Design review of the part shown in the three views and the two pictorial views. Dimensions are in mm from the part's minimum x, y and z. Give positions to 0.01 mm unless a question says otherwise; leave off trailing zeros. Write each loop counter-clockwise with the first axis right and the second up, starting at its lowest first coordinate (ties: lowest second). Pieces come first, ordered by that corner, then holes. Notation, with made-up numbers: (43.25, 44) -> (72.25, 44) arc R29 cw to (72.25, 73) -> close; hole circle Ø11 at (-39.5, 10.25). An arc over 180 degrees is marked (long way). Return JSON: item names as keys, results as strings. Group by question number.
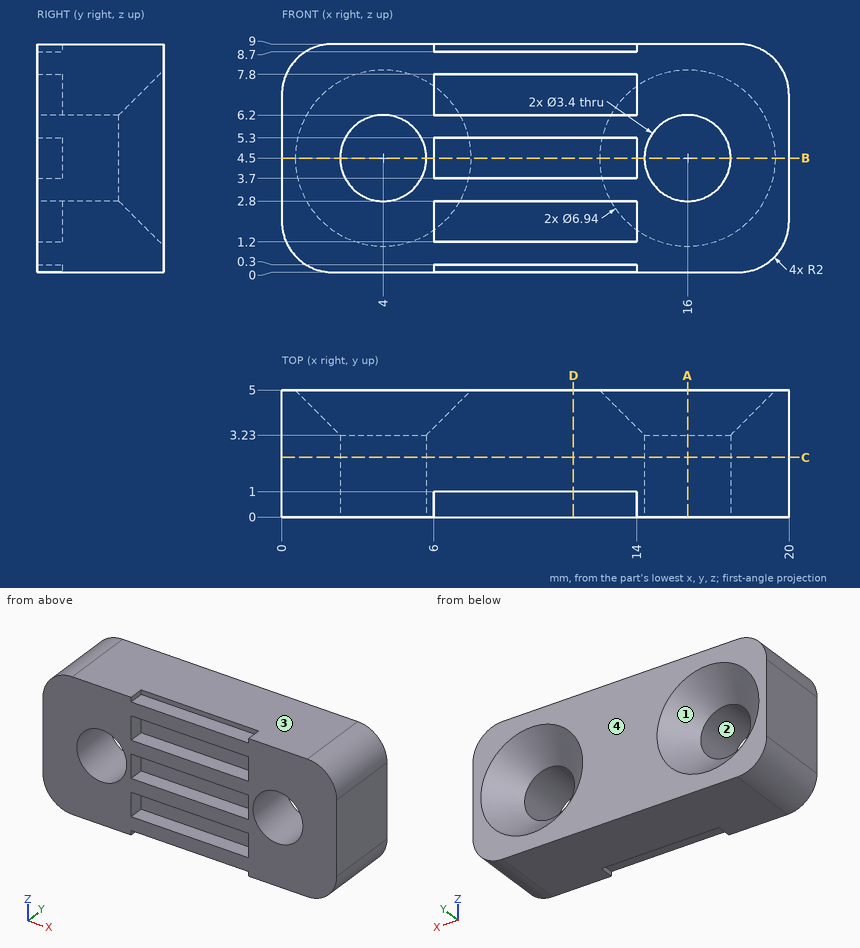
Q1. Take a section at C-C, the plane y = 2.35. Give the boundary of the cut face in (x, z).
Q2. Take a section at B-B, the plane z = 4.5. Give the boundary of the cut face in (x, y).
Q3. Take a section at D-D, the plane x = 11.5. Give the boundary of the cut face in (y, z).
Q4. Take a section at A-A, the plane x = 16. Give the boundary of the cut face in (y, z).
Q5. For L1, parallel to X at y = 2.1, z = 4.5; L2, parallel to Z at x = 11.5, y = 0.4; L3, parallel to X at y = 4, z = 3.5, list the stretches that pass through material, from the lowest coordinate up. Write a range as from..to.
Q6. Mouldability with a two-part tool opening along Z and no side actions: class the marked faces 1, 2, 3 and 4 as +Z half, -Z half, draft (parallel to the pull), parting line (faces both ways), or undercut.
Q7. Insertion check: pin 1 (4.5 mm diameter, centred on x = 16, z = 4.5, fed in from -Y); pin 2 (0.8 mm diameter, centred on x = 9.5, y = 0.5, fed in from +Z); pin 3 (2.5 mm diameter, centred on x = 4, z = 4.5, fed in from -Y); pin 4 (0.8 mm diameter, centred on x = 8, y = 0.5, fed in from -Z). Each pin has a flat end and moves straight along its axis. Give the tip position at first contact, or say it passes through.
Final values:
{
 "1": {"outline": "(0, 2) arc R2 ccw to (2, 0) -> (18, 0) arc R2 ccw to (20, 2) -> (20, 7) arc R2 ccw to (18, 9) -> (2, 9) arc R2 ccw to (0, 7) -> close; hole circle Ø3.4 at (4, 4.5); hole circle Ø3.4 at (16, 4.5)"},
 "2": {"outline": "(0, 0) -> (2.3, 0) -> (2.3, 3.23) -> (0.53, 5) -> (0, 5) -> close; (5.7, 0) -> (6, 0) -> (6, 1) -> (14, 1) -> (14, 0) -> (14.3, 0) -> (14.3, 3.23) -> (12.53, 5) -> (7.47, 5) -> (5.7, 3.23) -> close; (17.7, 0) -> (20, 0) -> (20, 5) -> (19.47, 5) -> (17.7, 3.23) -> close"},
 "3": {"outline": "(0, 0.3) -> (1, 0.3) -> (1, 0) -> (5, 0) -> (5, 9) -> (1, 9) -> (1, 8.7) -> (0, 8.7) -> (0, 7.8) -> (1, 7.8) -> (1, 6.2) -> (0, 6.2) -> (0, 5.3) -> (1, 5.3) -> (1, 3.7) -> (0, 3.7) -> (0, 2.8) -> (1, 2.8) -> (1, 1.2) -> (0, 1.2) -> close"},
 "4": {"outline": "(0, 0) -> (5, 0) -> (5, 1.03) -> (3.23, 2.8) -> (0, 2.8) -> close; (0, 6.2) -> (3.23, 6.2) -> (5, 7.97) -> (5, 9) -> (0, 9) -> close"},
 "5": {"L1": "x = 0..2.3, 5.7..14.3, 17.7..20", "L2": "z = 0.3..1.2, 2.8..3.7, 5.3..6.2, 7.8..8.7", "L3": "x = 0..1.74, 6.26..13.74, 18.26..20"},
 "6": {"face 1": "undercut", "face 2": "undercut", "face 3": "+Z half", "face 4": "draft"},
 "7": {"pin 1": "stops at y = 0", "pin 2": "stops at z = 8.7", "pin 3": "passes through", "pin 4": "stops at z = 0.3"}
}
